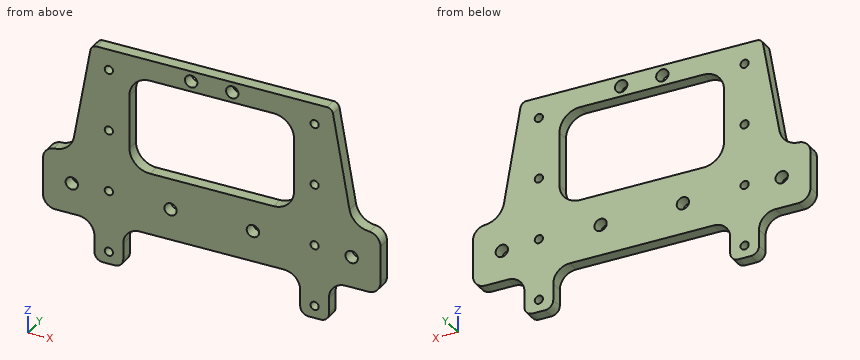
from build123d import *

# Parameters (mm, degrees)
SKETCH_1_R      = 1
SKETCH_1_R_2    = 1.5
EXTRUDE_1_DEPTH = 3


with BuildPart() as part:
    # 草图1 → 凸台-拉伸1 (new body)
    with BuildSketch(Plane(origin=(0, 0, 0), x_dir=(1, 0, 0), z_dir=(0, 1, 0))):
        with BuildLine():
            Line((-28.5, -2), (-28.5, -6))
            ThreePointArc((-28.5, -6), (-29.671572875, -8.828427125), (-32.5, -10))
            Line((-32.5, -10), (-38, -10))
            ThreePointArc((-38, -10), (-40.121320344, -10.878679656), (-41, -13))
            Line((-41, -13), (-41, -22))
            ThreePointArc((-41, -22), (-40.121320344, -24.121320344), (-38, -25))
            Line((-38, -25), (-38.391303062, -25))
            ThreePointArc((-38.391303062, -25), (-35.177365014, -26.169777784), (-33.467264297, -29.131759112))
            Line((-33.467264297, -29.131759112), (-29.47721163, -51.760472267))
            ThreePointArc((-29.47721163, -51.760472267), (-28.964181415, -52.649066665), (-28, -53))
            Line((-28, -53), (-22, -53))
            Line((-22, -53), (22, -53))
            Line((22, -53), (28, -53))
            ThreePointArc((28, -53), (28.964181415, -52.649066665), (29.47721163, -51.760472267))
            Line((29.47721163, -51.760472267), (33.467264297, -29.131759112))
            ThreePointArc((33.467264297, -29.131759112), (35.177365014, -26.169777784), (38.391303062, -25))
            Line((38.391303062, -25), (38, -25))
            ThreePointArc((38, -25), (40.121320344, -24.121320344), (41, -22))
            Line((41, -22), (41, -13))
            ThreePointArc((41, -13), (40.121320344, -10.878679656), (38, -10))
            Line((38, -10), (32.5, -10))
            ThreePointArc((32.5, -10), (29.671572875, -8.828427125), (28.5, -6))
            Line((28.5, -6), (28.5, -2))
            ThreePointArc((28.5, -2), (27.914213562, -0.585786438), (26.5, 0))
            Line((26.5, 0), (23.5, 0))
            ThreePointArc((23.5, 0), (22.085786438, -0.585786438), (21.5, -2))
            Line((21.5, -2), (21.5, -6))
            ThreePointArc((21.5, -6), (20.328427125, -8.828427125), (17.5, -10))
            Line((17.5, -10), (-17.5, -10))
            ThreePointArc((-17.5, -10), (-20.328427125, -8.828427125), (-21.5, -6))
            Line((-21.5, -6), (-21.5, -2))
            ThreePointArc((-21.5, -2), (-22.085786438, -0.585786438), (-23.5, 0))
            Line((-23.5, 0), (-26.5, 0))
            ThreePointArc((-26.5, 0), (-27.914213562, -0.585786438), (-28.5, -2))
        make_face()
        with Locations(Location((-25, -48, 0), (0, 0, 270))):
            Circle(SKETCH_1_R, mode=Mode.SUBTRACT)
        with Locations(Location((-25, -33, 0), (0, 0, 270))):
            Circle(SKETCH_1_R, mode=Mode.SUBTRACT)
        with Locations(Location((-25, -18, 0), (0, 0, 270))):
            Circle(SKETCH_1_R, mode=Mode.SUBTRACT)
        with Locations(Location((-34, -17.5, 0), (0, 0, 270))):
            Circle(SKETCH_1_R_2, mode=Mode.SUBTRACT)
        with Locations(Location((-10, -17.5, 0), (0, 0, 270))):
            Circle(SKETCH_1_R_2, mode=Mode.SUBTRACT)
        with Locations(Location((10, -17.5, 0), (0, 0, 270))):
            Circle(SKETCH_1_R_2, mode=Mode.SUBTRACT)
        with Locations(Location((34, -17.5, 0), (0, 0, 270))):
            Circle(SKETCH_1_R_2, mode=Mode.SUBTRACT)
        with Locations(Location((25, -18, 0), (0, 0, 270))):
            Circle(SKETCH_1_R, mode=Mode.SUBTRACT)
        with Locations(Location((25, -33, 0), (0, 0, 270))):
            Circle(SKETCH_1_R, mode=Mode.SUBTRACT)
        with Locations(Location((25, -48, 0), (0, 0, 270))):
            Circle(SKETCH_1_R, mode=Mode.SUBTRACT)
        with Locations(Location((-25, -3, 0), (0, 0, 270))):
            Circle(SKETCH_1_R, mode=Mode.SUBTRACT)
        with Locations(Location((25, -3, 0), (0, 0, 270))):
            Circle(SKETCH_1_R, mode=Mode.SUBTRACT)
        with Locations(Location((5, -50.5, 0), (0, 0, 270))):
            Circle(SKETCH_1_R_2, mode=Mode.SUBTRACT)
        with Locations(Location((-5, -50.5, 0), (0, 0, 270))):
            Circle(SKETCH_1_R_2, mode=Mode.SUBTRACT)
        with BuildLine():
            Line((-20, -43), (-20, -30))
            ThreePointArc((-20, -30), (-18.535533906, -26.464466094), (-15, -25))
            Line((-15, -25), (15, -25))
            ThreePointArc((15, -25), (18.535533906, -26.464466094), (20, -30))
            Line((20, -30), (20, -43))
            ThreePointArc((20, -43), (18.535533906, -46.535533906), (15, -48))
            Line((15, -48), (-15, -48))
            ThreePointArc((-15, -48), (-18.535533906, -46.535533906), (-20, -43))
        make_face(mode=Mode.SUBTRACT)
    extrude(amount=EXTRUDE_1_DEPTH)


solid = part.part
Part model, mm, in its own coordinate system. Coordinates: 2 decimals unless noted, no trailing zeros. Order: outer loops, then holes, each group sorted by start corner. A loop starts at its lowest first (then second) coordinate and runs counter-clockwise, first axis right, second up. Notation, with made-up numbers: M 17,76.5 L 71,76.5 A19 ccw 71,90.5 Z; hole C -7.5,65.5 d9. An arc over 180 degrees is marked long. One line per question, with ' | ' between items.
Q1. Slice it at A-A (x = 5). Give the cut face in (y, z).
A:
outline: M 0,10 L 3,10 L 3,25 L 0,25 Z; M 0,48 L 3,48 L 3,49 L 0,49 Z; M 0,52 L 3,52 L 3,53 L 0,53 Z
Q2. Slice it at C-C (z = 33). Give the cut face in (x, y).
A:
outline: M -32.79,0 L -26,0 L -26,3 L -32.79,3 Z; M -24,0 L -20,0 L -20,3 L -24,3 Z; M 20,0 L 24,0 L 24,3 L 20,3 Z; M 26,0 L 32.79,0 L 32.79,3 L 26,3 Z
Q3. Pin check, flat tips, straight feed: P1, Ø1.2, axis at x = -25, z = 48, coming from the -Y side; P2, Ø1.5, axis at y = 1.5, z = 3.5, coming from the -X side; P3, Ø1.5, axis at x = -32, y = 2, coming from the -Z side; P4, Ø0.9, axis at y = 1, z = 4, coming from the +X side. Stop position of each tip, or through.
A:
P1: passes through | P2: stops at x = -28.5 | P3: stops at z = 9.8 | P4: stops at x = 28.5
Q4. Drill centre lines: line 1 (X direction, y = 1.3, z = 3); line 2 (X direction, y = 2.3, z = 5); line 3 (X direction, y = 2.2, z = 50.5). Where is each one in solid material? Low to high.
A:
line 1: x = -28.5 to -26, -24 to -21.5, 21.5 to 24, 26 to 28.5 | line 2: x = -28.5 to -21.5, 21.5 to 28.5 | line 3: x = -29.7 to -6.5, -3.5 to 3.5, 6.5 to 29.7
Q5. Slice it at D-D (z = 38.5). Give the cut face in (x, y).
A:
outline: M -31.82,0 L -20,0 L -20,3 L -31.82,3 Z; M 20,0 L 31.82,0 L 31.82,3 L 20,3 Z
Q6. Slice it at B-B (z = 50.5). Give the cut face in (x, y).
A:
outline: M -29.7,0 L -6.5,0 L -6.5,3 L -29.7,3 Z; M -3.5,0 L 3.5,0 L 3.5,3 L -3.5,3 Z; M 6.5,0 L 29.7,0 L 29.7,3 L 6.5,3 Z
